Here's how the part is built. I have some questions about the finished solid (model axes, mm). Coordinates: 2 decimals unless noted, no trailing zeros. Write each loop counter-clockwise with the first axis right and the second up, starting at its lowest first coordinate (ties: lowest second). Pieces come first, ordered by that corner, then holes. Notation, with made-up numbers: (-36.75, 47) -> (-15.75, 47) arc R25 cw to (-15.75, 82) -> close; hole circle Ø8 at (18, 57). An arc over 180 degrees is marked (long way). Put each result on its own line as item: value. Start each with the question number.
Item 1: If we mould it in two halves opening along Y, with no side actions, what happens to faces 1 (the face through (-1, 38, 1)), 2 (the face through (-1, -38, 1)), 3 (the face through (26.736, -26.966, 1.521)), 4 (the face through (38, -1, 1))? For each: released by +Y, released by -Y, zero draft, split by the parting line, or undercut.
Item 2: For pin 1 (10 mm diameter, centred on x = -13, y = 21.5, fed in from -Z); pin 2 (1.5 mm diameter, centred on x = 17, y = 20.5, fed in from +Z), each with a flat end and sliding along its axis, tell me the tip position at first contact or that it passes through.
Item 3: I want a section at C-C, the plane z = 2.55. State how many separate pieces and enclosed holes the cut face has, then the cut area to 3 significant figures.
Item 4: I need wall thicknesses on line 1 (X direction, y = 22, z = 2); line 2 (Y direction, x = 29.5, z = 1.75); line 3 (Y direction, x = 18, z = 1.95). Which ranges of each line are inside material? Lowest first, please. Write a range as [from, to].
Item 5: I want a section at A-A, the plane x = 1.5. List the corners of the cut face in (y, z) for me, then the cut area to 3 significant figures.
Item 6: I want a section at B-B, the plane y = -29.5. List the corners of the cut face in (x, z) for me, then the cut area to 3 significant figures.
from build123d import *

# Parameters (mm, degrees)
F0_W     = 76
F0_H     = 76
F1_DEPTH = 3
F3_DEPTH = 25
F4_R     = 3.75
F5_DEPTH = 25


with BuildPart() as f1:
    # F0 (on Top) → F1 (new body)
    with BuildSketch(Plane.XY):
        Rectangle(F0_W, F0_H)
    extrude(amount=F1_DEPTH)

    # F2 (on face) → F3 (cut)
    with BuildSketch(Plane.XY.offset(3)):
        with BuildLine():
            ThreePointArc((24.9688578028, 11.5241546337), (23.0631205202, 7.4936621136), (26.9739584315, 5.3530894386))
            ThreePointArc((26.9739584315, 5.3530894386), (26.1540541981, 8.4979673453), (24.9688578028, 11.5241546337))
        make_face()
        with BuildLine():
            ThreePointArc((24.9688578028, 11.5241546337), (26.1540541981, 8.4979673453), (26.9739584315, 5.3530894386))
            ThreePointArc((26.9739584315, 5.3530894386), (28.7257451553, 6.5107819939), (29.4040541981, 8.4979673453))
            ThreePointArc((29.4040541981, 8.4979673453), (27.9858035963, 11.1825891329), (24.9688578028, 11.5241546337))
        make_face()
        with BuildLine():
            ThreePointArc((29.4040541981, -8.4979673453), (28.7257451553, -6.5107819939), (26.9739584315, -5.3530894386))
            ThreePointArc((26.9739584315, -5.3530894386), (26.1540541981, -8.4979673453), (24.9688578028, -11.5241546337))
            ThreePointArc((24.9688578028, -11.5241546337), (27.9858035963, -11.1825891329), (29.4040541981, -8.4979673453))
        make_face()
        with BuildLine():
            ThreePointArc((24.9688578028, -11.5241546337), (26.1540541981, -8.4979673453), (26.9739584315, -5.3530894386))
            ThreePointArc((26.9739584315, -5.3530894386), (23.0631205202, -7.4936621136), (24.9688578028, -11.5241546337))
        make_face()
        with BuildLine():
            ThreePointArc((13.4265021538, 23.9995633276), (14.2537923681, 19.6186621136), (18.6759237504, 20.1856352902))
            ThreePointArc((18.6759237504, 20.1856352902), (16.164094438, 22.2479673453), (13.4265021538, 23.9995633276))
        make_face()
        with BuildLine():
            ThreePointArc((13.4265021538, 23.9995633276), (16.164094438, 22.2479673453), (18.6759237504, 20.1856352902))
            ThreePointArc((18.6759237504, 20.1856352902), (19.2239919253, 21.1527379778), (19.414094438, 22.2479673453))
            ThreePointArc((19.414094438, 22.2479673453), (17.0765978836, 25.3672360836), (13.4265021538, 23.9995633276))
        make_face()
        with BuildLine():
            ThreePointArc((19.414094438, -22.2479673453), (19.2239919253, -21.1527379778), (18.6759237504, -20.1856352902))
            ThreePointArc((18.6759237504, -20.1856352902), (16.164094438, -22.2479673453), (13.4265021538, -23.9995633276))
            ThreePointArc((13.4265021538, -23.9995633276), (17.0765978836, -25.3672360836), (19.414094438, -22.2479673453))
        make_face()
        with BuildLine():
            ThreePointArc((13.4265021538, -23.9995633276), (16.164094438, -22.2479673453), (18.6759237504, -20.1856352902))
            ThreePointArc((18.6759237504, -20.1856352902), (14.2537923681, -19.6186621136), (13.4265021538, -23.9995633276))
        make_face()
        with BuildLine():
            ThreePointArc((-3.244320968, 27.3079545455), (0, 24.25), (3.244320968, 27.3079545455))
            ThreePointArc((3.244320968, 27.3079545455), (0, 27.5), (-3.244320968, 27.3079545455))
        make_face()
        with BuildLine():
            ThreePointArc((-3.244320968, 27.3079545455), (0, 27.5), (3.244320968, 27.3079545455))
            ThreePointArc((3.244320968, 27.3079545455), (3.2485799318, 27.4039352978), (3.25, 27.5))
            ThreePointArc((3.25, 27.5), (-0.0960647022, 30.7485799318), (-3.244320968, 27.3079545455))
        make_face()
        with BuildLine():
            ThreePointArc((3.25, -27.5), (3.2485799318, -27.4039352978), (3.244320968, -27.3079545455))
            ThreePointArc((3.244320968, -27.3079545455), (0, -27.5), (-3.244320968, -27.3079545455))
            ThreePointArc((-3.244320968, -27.3079545455), (-0.0960647022, -30.7485799318), (3.25, -27.5))
        make_face()
        with BuildLine():
            ThreePointArc((-3.244320968, -27.3079545455), (0, -27.5), (3.244320968, -27.3079545455))
            ThreePointArc((3.244320968, -27.3079545455), (0, -24.25), (-3.244320968, -27.3079545455))
        make_face()
        with BuildLine():
            ThreePointArc((-12.914094438, 22.2479673453), (-13.0448256997, 23.1604707908), (-13.4265021538, 23.9995633276))
            ThreePointArc((-13.4265021538, 23.9995633276), (-16.164094438, 22.2479673453), (-18.6759237504, 20.1856352902))
            ThreePointArc((-18.6759237504, 20.1856352902), (-15.0688650706, 19.188069858), (-12.914094438, 22.2479673453))
        make_face()
        with BuildLine():
            ThreePointArc((-18.6759237504, 20.1856352902), (-16.164094438, 22.2479673453), (-13.4265021538, 23.9995633276))
            ThreePointArc((-13.4265021538, 23.9995633276), (-18.074396508, 24.877272577), (-18.6759237504, 20.1856352902))
        make_face()
        with BuildLine():
            ThreePointArc((-18.6759237504, -20.1856352902), (-18.074396508, -24.877272577), (-13.4265021538, -23.9995633276))
            ThreePointArc((-13.4265021538, -23.9995633276), (-16.164094438, -22.2479673453), (-18.6759237504, -20.1856352902))
        make_face()
        with BuildLine():
            ThreePointArc((-18.6759237504, -20.1856352902), (-16.164094438, -22.2479673453), (-13.4265021538, -23.9995633276))
            ThreePointArc((-13.4265021538, -23.9995633276), (-13.0448256997, -23.1604707908), (-12.914094438, -22.2479673453))
            ThreePointArc((-12.914094438, -22.2479673453), (-15.0688650706, -19.188069858), (-18.6759237504, -20.1856352902))
        make_face()
        with BuildLine():
            ThreePointArc((-22.9040541981, 8.4979673453), (-23.4694324105, 10.3297167435), (-24.9688578028, 11.5241546337))
            ThreePointArc((-24.9688578028, 11.5241546337), (-26.1540541981, 8.4979673453), (-26.9739584315, 5.3530894386))
            ThreePointArc((-26.9739584315, 5.3530894386), (-24.1668688467, 5.9262763881), (-22.9040541981, 8.4979673453))
        make_face()
        with BuildLine():
            ThreePointArc((-26.9739584315, 5.3530894386), (-26.1540541981, 8.4979673453), (-24.9688578028, 11.5241546337))
            ThreePointArc((-24.9688578028, 11.5241546337), (-29.2449878761, 9.502272577), (-26.9739584315, 5.3530894386))
        make_face()
        with BuildLine():
            ThreePointArc((-26.9739584315, -5.3530894386), (-29.2449878761, -9.502272577), (-24.9688578028, -11.5241546337))
            ThreePointArc((-24.9688578028, -11.5241546337), (-26.1540541981, -8.4979673453), (-26.9739584315, -5.3530894386))
        make_face()
        with BuildLine():
            ThreePointArc((-26.9739584315, -5.3530894386), (-26.1540541981, -8.4979673453), (-24.9688578028, -11.5241546337))
            ThreePointArc((-24.9688578028, -11.5241546337), (-23.4694324105, -10.3297167435), (-22.9040541981, -8.4979673453))
            ThreePointArc((-22.9040541981, -8.4979673453), (-24.1668688467, -5.9262763881), (-26.9739584315, -5.3530894386))
        make_face()
    extrude(amount=-F3_DEPTH, mode=Mode.SUBTRACT)

    # F4 (on face) → F5 (cut)
    with BuildSketch(Plane.XY.offset(3)):
        with Locations((29.5, -29.5)):
            Circle(F4_R)
    extrude(amount=-F5_DEPTH, mode=Mode.SUBTRACT)


solid = f1.part
Calculated:
1. face 1: released by +Y
1. face 2: released by -Y
1. face 3: undercut
1. face 4: zero draft
2. pin 1: stops at z = 0
2. pin 2: passes through
3. separate pieces: 1
3. enclosed holes: 11
3. area: 5,400 mm2
4. line 1: x = [-38, -19.4], [-12.92, 12.92], [19.4, 38]
4. line 2: y = [-38, -33.25], [-25.75, 38]
4. line 3: y = [-38, -24.93], [-19.57, 19.57], [24.93, 38]
5. outline: (-38, 0) -> (-30.38, 0) -> (-30.38, 3) -> (-38, 3) -> close; (-24.62, 0) -> (24.62, 0) -> (24.62, 3) -> (-24.62, 3) -> close; (30.38, 0) -> (38, 0) -> (38, 3) -> (30.38, 3) -> close
5. area: 193 mm2
6. outline: (-38, 0) -> (-2.56, 0) -> (-2.56, 3) -> (-38, 3) -> close; (2.56, 0) -> (25.75, 0) -> (25.75, 3) -> (2.56, 3) -> close; (33.25, 0) -> (38, 0) -> (38, 3) -> (33.25, 3) -> close
6. area: 190 mm2
